```python
from build123d import *

# Parameters (mm, degrees)
EXTRUDE1_DEPTH      = 28.448
EXTRUDE1_DEPTH_BACK = 28.448
SKETCH7_R           = 20.066
EXTRUDE2_DEPTH      = 731.393
SKETCH8_R           = 34.173782646
EXTRUDE3_DEPTH      = 60.96
SKETCH9_R           = 19.812
EXTRUDE4_DEPTH      = 60.96


with BuildPart() as part:
    # Sketch6 → Extrude1 (new body, two sides)
    with BuildSketch(Plane(origin=(0, 0, 0), x_dir=(0, 0, -1), z_dir=(1, 0, 0))) as extrude1_sk:
        with BuildLine():
            Line((36.538920518, 71.697598607), (-36.538913711, 71.697596168))
            ThreePointArc((-36.538913711, 71.697596168), (-37.054496025, 70.591976021), (-37.3703, 69.41363444))
            Line((-37.3703, 69.41363444), (-48.25031, 7.73618444))
            ThreePointArc((-48.25031, 7.73618444), (5e-06, -49.77053593), (48.25032, 7.73618444))
            Line((48.25032, 7.73618444), (37.37031, 69.41363444))
            ThreePointArc((37.37031, 69.41363444), (37.054505048, 70.591977567), (36.538920518, 71.697598607))
        make_face()
    extrude(amount=EXTRUDE1_DEPTH)
    extrude(extrude1_sk.sketch, amount=-EXTRUDE1_DEPTH_BACK)

    # Sketch7 → Extrude2 (add)
    with BuildSketch(Plane(origin=(0, 71.697597388, 2.392e-06), x_dir=(-1, 0, 0), z_dir=(0, 1, 3.3e-08))):
        Circle(SKETCH7_R)
    extrude(amount=EXTRUDE2_DEPTH)

    # Sketch8 → Extrude3 (add)
    with BuildSketch(Plane(origin=(28.448, 0, 0), x_dir=(0, 0, -1), z_dir=(1, 0, 0))):
        Circle(SKETCH8_R)
    extrude(amount=-EXTRUDE3_DEPTH)

    # Sketch9 → Extrude4 (add)
    with BuildSketch(Plane(origin=(28.448, 0, 0), x_dir=(0, 0, -1), z_dir=(1, 0, 0))):
        Circle(SKETCH9_R)
    extrude(amount=EXTRUDE4_DEPTH)


solid = part.part
```
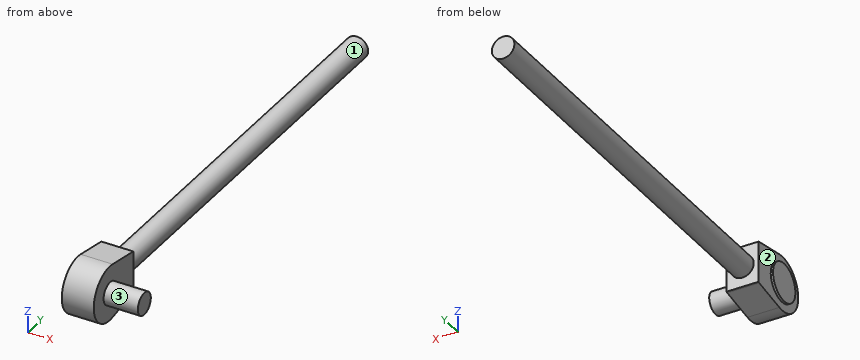
CAD build for the part. Positions are in the model's coordinates, mm. Face numbers are marked on the shaded views. A direction names the side the tool comes from. Round coordinates to 2 decimals unless told otherwise and drop trailing zeros. Write each loop counter-clockwise with the first axis right and the second up, starting at its lowest first coordinate (ties: lowest second). Pieces come first, ordered by that corner, then holes. Notation, with made-up numbers: (-34.75, 5.5) -> (-19.75, 5.5) arc R33 ccw to (-19.75, 33.5) -> close; hole circle Ø6 at (-6, 45). An arc over 180 degrees is marked (long way). Answer in a Markdown table with one row per item. Add a question column.
Item 1: Saw through at B-B, the plane y = 0. Write the cut outline in (x, z).
Item 2: Saw through at A-A, the plane x = 0. Write the cut outline in (y, z), then the cut area to 3 significant figures.
Item 3: Saw through at C-C, the plane x = 79. Write the cut outline in (y, z).
Item 4: Which spindle directions (+Z, -Z, +X, -X, +Y, -Y) get a long thin tool onto all of the face, cutting with end or side? Do the marked faces 1, 2 and 3. Say none if no direction does.
Item 5: Drop flat-ended pins along their axis: pin 1 Ø5 at (x, z) = (27.5, 27.5) entering from +Y; pin 2 Ø6 at (x, z) = (-20, -6.5) entering from -Y; pin 3 Ø4 at (y, z) = (226.5, -17) entering from +X. Give the stop position or say it passes through.
Item 6: Drill centre lines: line 1 (Z direction, x = 0.5, y = 541.5); line 2 (X direction, y = 486.5, z = -3); line 3 (Y direction, x = 70.5, z = 2). Where is each one in solid material? Low to high. Write a range as from..to.
Findings below:
| question | item | result |
|---|---|---|
| 1 | outline | (-32.51, -34.17) -> (-28.45, -34.17) -> (-28.45, -48.99) -> (28.45, -48.99) -> (28.45, -19.81) -> (89.41, -19.81) -> (89.41, 19.81) -> (28.45, 19.81) -> (28.45, 48.99) -> (-28.45, 48.99) -> (-28.45, 34.17) -> (-32.51, 34.17) -> close |
| 2 | outline | (7.74, -48.25) -> (69.41, -37.37) arc R7 ccw to (71.7, -36.54) -> (71.7, -20.07) -> (803.09, -20.07) -> (803.09, 20.07) -> (71.7, 20.07) -> (71.7, 36.54) arc R7 ccw to (69.41, 37.37) -> (7.74, 48.25) arc R49 ccw (long way) to start |
| 2 | area | 39,400 mm^2 |
| 3 | outline | circle Ø39.62 at (0, 0) |
| 4 | face 1 | +Y |
| 4 | face 2 | -X |
| 4 | face 3 | +X |
| 5 | pin 1 | stops at y = 71.7 |
| 5 | pin 2 | stops at y = -49.65 |
| 5 | pin 3 | stops at x = 13.33 |
| 6 | line 1 | z = -20.06..20.06 |
| 6 | line 2 | x = -19.84..19.84 |
| 6 | line 3 | y = -19.71..19.71 |
